from build123d import *

# Parameters (mm, degrees)
F0_W     = 5.6
F0_H     = 10
F1_DEPTH = 7
F2_DEPTH = 1.58
F4_DEPTH = 3


with BuildPart() as f1:
    # F0 (on Top) → F1 (new body)
    with BuildSketch(Plane.XY):
        with Locations((-16.725898, -1.059211)):
            Rectangle(F0_W, F0_H)
        Polygon((8.174102, 3.940789), (5.374102, 3.940789), (2.574102, 3.940789), (2.574102, -6.059211), (8.174102, -6.059211), align=None)
        with Locations((27.474102, -1.059211)):
            Rectangle(F0_W, F0_H)
    extrude(amount=-F1_DEPTH)

    # F0 (on Top) → F2 (join)
    with BuildSketch(Plane.XY):
        Polygon((33.174102, 5.940789), (-22.425898, 5.940789), (-27.725898, 0.940789), (-27.725898, -18.059211), (38.474102, -18.059211), (38.474102, 0.940789), align=None)
        with Locations((-16.725898, -1.059211)):
            Rectangle(F0_W, F0_H, mode=Mode.SUBTRACT)
        Polygon((2.574102, 3.940789), (5.374102, 3.940789), (8.174102, 3.940789), (8.174102, -6.059211), (2.574102, -6.059211), align=None, mode=Mode.SUBTRACT)
        with Locations((27.474102, -1.059211)):
            Rectangle(F0_W, F0_H, mode=Mode.SUBTRACT)
        with Locations((-16.725898, -1.059211)):
            Rectangle(F0_W, F0_H)
        Polygon((8.174102, 3.940789), (5.374102, 3.940789), (2.574102, 3.940789), (2.574102, -6.059211), (8.174102, -6.059211), align=None)
        with Locations((27.474102, -1.059211)):
            Rectangle(F0_W, F0_H)
    extrude(amount=F2_DEPTH)

    # F3 (on face) → F4 (join)
    with BuildSketch(Plane.XY.offset(1.58)):
        Polygon((-1.125898, -18.059211), (5.374102, -18.059211), (11.874102, -18.059211), (11.874102, -15.659211), (-1.125898, -15.659211), align=None)
    extrude(amount=F4_DEPTH)


solid = f1.part
Verification items for the finished model (mm, model axes). A direction names the side the tool comes from. Coordinates: 2 decimals unless noted, no trailing zeros. Order: outer loops, then holes, each group sorted by start corner. A loop starts at its lowest first (then second) coordinate and runs counter-clockwise, first axis right, second up.
Item 1: Section check A-A, the plane z = -3. Enter the section's corners in (x, y), then the cut area to 3 significant figures.
Filled in:
outline: (-19.53, -6.06) - (-13.93, -6.06) - (-13.93, 3.94) - (-19.53, 3.94) - close; (2.57, -6.06) - (8.17, -6.06) - (8.17, 3.94) - (2.57, 3.94) - close; (24.67, -6.06) - (30.27, -6.06) - (30.27, 3.94) - (24.67, 3.94) - close
area: 168 mm2
Item 2: Section check C-C, the plane x = 4.5. Enter the section's corners in (y, z).
Filled in:
outline: (-18.06, 0) - (-6.06, 0) - (-6.06, -7) - (3.94, -7) - (3.94, 0) - (5.94, 0) - (5.94, 1.58) - (-15.66, 1.58) - (-15.66, 4.58) - (-18.06, 4.58) - close
Item 3: Section check B-B, the plane y = -2.5. Enter the section's corners in (x, z).
Filled in:
outline: (-27.73, 0) - (-19.53, 0) - (-19.53, -7) - (-13.93, -7) - (-13.93, 0) - (2.57, 0) - (2.57, -7) - (8.17, -7) - (8.17, 0) - (24.67, 0) - (24.67, -7) - (30.27, -7) - (30.27, 0) - (38.47, 0) - (38.47, 1.58) - (-27.73, 1.58) - close
Item 4: Material ranges on L1, parallel to X at y = 1, z = -6.25; L2, parallel to Z at x = -6, y = 2; L3, parallel to Z at x = 10.5, y = -16.75, recorded low to high.
Filled in:
L1: x = -19.53 to -13.93, 2.57 to 8.17, 24.67 to 30.27
L2: z = 0 to 1.58
L3: z = 0 to 4.58
Item 5: Release check for a two-part mould opening along X. For faces 4 (the face through (38.474, -9, 1)), 5 (the face through (24.674, -1, -3)), 6 (the face through (27, -1, -7)) record: +X half, -X half, draft (parallel to the pull), parting line (faces both ways), or undercut.
Filled in:
face 4: +X half
face 5: undercut
face 6: draft
Item 6: Depth check by flat-ended pin: pin 1 (1 mm diameter, centred on x = 10.5, y = 1, fed in from -Z); pin 2 (4.5 mm diameter, centred on x = -15.5, z = -5, fed in from +Y); pin 3 (2 mm diameter, centred on y = -0.5, z = -2, fed in from -X). Enter the tip coordinate at first touch or a pass-through.
Filled in:
pin 1: stops at z = 0
pin 2: stops at y = 3.94
pin 3: stops at x = -19.53
Item 7: Access from +Z, -Z, +X, -X, +Y, -Y to the whole of each face (thin tool, end or side, straight path). Record for faces 1 (the face through (-1.126, -17, 3)), 2 (the face through (8.174, -1, -3)), 3 (the face through (-17, 3.941, -3)).
Filled in:
face 1: +Z, -X, +Y, -Y
face 2: -Z, +Y, -Y
face 3: -Z, +X, -X, +Y
Item 8: Section check D-D, the plane z = 0.75. Enter the section's corners in (x, y).
Filled in:
outline: (-27.73, -18.06) - (38.47, -18.06) - (38.47, 0.94) - (33.17, 5.94) - (-22.43, 5.94) - (-27.73, 0.94) - close
